Input: part model. Units: mm. Frame: model coordinates. A direction names the side the tool comes from. Give positions to 0.01 mm unless a question says otherwise; leave off trailing zeros. Write each loop counter-clockwise with the first axis right and the second up, starting at its lowest first coordinate (ties: lowest second). Pieces come first, ordered by that corner, then holes. Notation, with made-up numbers: (-13, 48) -> (24, 48) arc R21 ccw to (24, 63) -> close; hole circle Ø3 at (-28.75, 13.25). An arc over 180 degrees is marked (long way). Return JSON: item names as keys, results as strings. Group by question number.
Item 1: Line query: line 1 (X direction, y = 1, z = 1.45); line 2 (Y direction, x = -25.5, z = 2.1); line 3 (X direction, y = 43.5, z = 0.35). Output: solid intervals per line, ascending. Write a range as [from, to].
Item 2: Set-up query: faces 5 (the face through (2, 49, 2)), 6 (the face through (30.595, 53, 2)). Return all of +Z, -Z, +X, -X, +Y, -Y with unobstructed straight access to the full face (end or side cutting, diameter ignored); none if empty.
Item 3: Pin query (flat end, axial travel): P1, Ø13, axis at x = -25.04, y = 47.63, coming from the +Z side. Return the tip coordinate at first contact, or that it passes through.
Item 4: Section C-C, the plane z = 1.4. Return loops of the section in (x, y).
Item 5: Mould query, pull axis Y, two halves, no side actions, for faces 1 (the face through (0, 51, 2)), 2 (the face through (-3, -12.985, 2)), 3 (the face through (-4, 53, 0)), 4 (the face through (-26.82, 55.65, 1.57)). Classes: released by +Y, released by -Y, zero draft, split by the parting line, or undercut.
Item 6: Section B-B, the plane y = 83. Return loops of the section in (x, z), then the cut area to 3 significant figures.
Item 7: Section A-A, the plane x = -22. Return loops of the section in (y, z).
Autodesk Fusion 360 part; units mm, degrees
sketch "Sketch1" plane through (0, 0, 0) normal (0, 0, 1) x (1, 0, 0)
  line L0 (0, 114) -> (2, 114)
  line L1 (2, 0) -> (0, 0)
  line L2 (30.5953, -12.9847) -> (-37.9542, -12.9847)
  line L3 (-37.9542, -12.9847) -> (-37.9542, 117.0153)
  line L4 (-37.9542, 117.0153) -> (30.5953, 117.0153)
  line L5 (30.5953, 117.0153) -> (30.5953, -12.9847)
  line L6 (0, 0) -> (2, 0)
  line L7 (2, 0) -> (2, 100)
  line L8 (2, 100) -> (0, 100)
  line L9 (0, 100) -> (0, 0)
  circle A0 centre (-25.0399, 47.6257) radius 8.2184
  dimension "d2" = 2
  dimension "d5" = 68.5495
  dimension "d8" = 2
  dimension "d9" = 100
  dimension "d10" = 130
  dimension "d19" = 16.4367
extrude "Extrude7" add sketch "Sketch1" along normal blind 3.176
Answer below:
{
 "1": {"line 1": "x = [-37.95, 0], [2, 30.6]", "line 2": "y = [-12.98, 39.42], [55.83, 117.02]", "line 3": "x = [-37.95, -32.15], [-17.93, 0], [2, 30.6]"},
 "2": {"face 5": "+Z, -Z", "face 6": "+Z, -Z, +X, +Y, -Y"},
 "3": {"P1": "passes through"},
 "4": {"outline": "(-37.95, -12.98) -> (30.6, -12.98) -> (30.6, 117.02) -> (-37.95, 117.02) -> close; hole circle Ø16.44 at (-25.04, 47.63); hole (0, 0) -> (2, 0) -> (2, 100) -> (0, 100) -> close"},
 "5": {"face 1": "undercut", "face 2": "released by -Y", "face 3": "zero draft", "face 4": "undercut"},
 "6": {"outline": "(-37.95, 0) -> (0, 0) -> (0, 3.18) -> (-37.95, 3.18) -> close; (2, 0) -> (30.6, 0) -> (30.6, 3.18) -> (2, 3.18) -> close", "area": "211 mm2"},
 "7": {"outline": "(-12.98, 0) -> (39.99, 0) -> (39.99, 3.18) -> (-12.98, 3.18) -> close; (55.26, 0) -> (117.02, 0) -> (117.02, 3.18) -> (55.26, 3.18) -> close"}
}
